Verification items for this drawing (mm, ordinates from the low corner). Give positions to 0.01 mm unless a question says otherwise; leave off trailing zeros. Write each loop counter-clockwise with the first axis right and the second up, starting at its lowest first coordinate (ties: lowest second). Pieces come first, ordered by that corner, then holes. Notation, with made-up numbers: (34.5, 43) -> (82.5, 43) arc R30 cw to (82.5, 70) -> close; hole circle Ø2 at (-21.5, 7). An arc over 180 degrees is marked (long way). Answer as a JSON object with one key per item and string values.
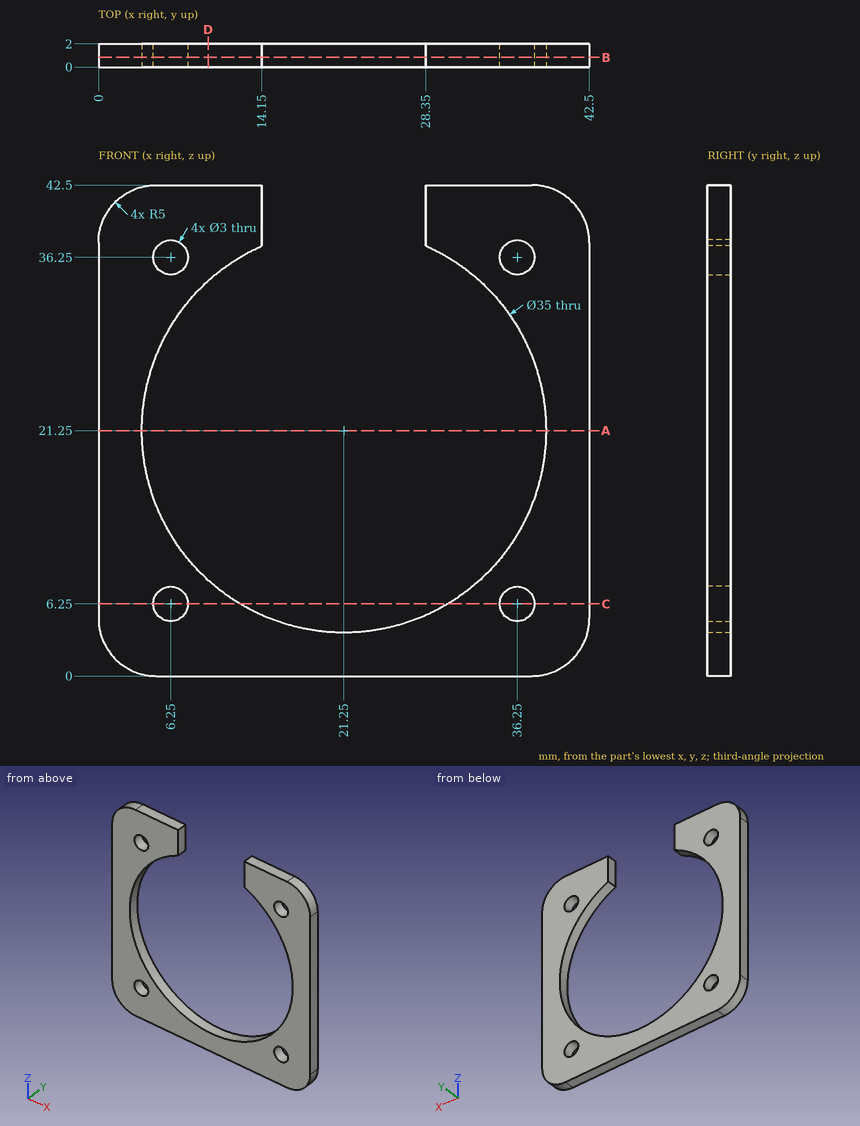
1. Sectioned sample at C-C, the plane z = 6.25. Enter the section's corners in (x, y).
Determined:
{"outline": "(0, 0) -> (4.75, 0) -> (4.75, 2) -> (0, 2) -> close; (7.75, 0) -> (12.24, 0) -> (12.24, 2) -> (7.75, 2) -> close; (30.26, 0) -> (34.75, 0) -> (34.75, 2) -> (30.26, 2) -> close; (37.75, 0) -> (42.5, 0) -> (42.5, 2) -> (37.75, 2) -> close"}
2. Go/stop test with flat-tipped pins: P1, Ø1, axis at y = 1.5, z = 39.5, coming from the +X side; P2, Ø1, axis at x = 17.5, y = 1, coming from the +Z side; P3, Ø1, axis at y = 1, z = 40.5, coming from the -X side. Record where each tip stops, or that it passes through.
Determined:
{"P1": "x = 42.27", "P2": "z = 4.27", "P3": "x = 0.67"}
3. Sectioned sample at A-A, the plane z = 21.25. Enter the section's corners in (x, y), plus the area to 3 significant figures.
Determined:
{"outline": "(0, 0) -> (3.75, 0) -> (3.75, 2) -> (0, 2) -> close; (38.75, 0) -> (42.5, 0) -> (42.5, 2) -> (38.75, 2) -> close", "area": "15.0 mm^2"}
4. Sectioned sample at B-B, the plane y = 0.85. Enter the section's corners in (x, z) (3 decimals).
Determined:
{"outline": "(0, 5) arc R5 ccw to (5, 0) -> (37.5, 0) arc R5 ccw to (42.5, 5) -> (42.5, 37.5) arc R5 ccw to (37.5, 42.5) -> (28.35, 42.5) -> (28.35, 37.245) arc R17.5 cw (long way) to (14.15, 37.245) -> (14.15, 42.5) -> (5, 42.5) arc R5 ccw to (0, 37.5) -> close; hole circle Ø3 at (6.25, 6.25); hole circle Ø3 at (6.25, 36.25); hole circle Ø3 at (36.25, 6.25); hole circle Ø3 at (36.25, 36.25)"}
5. Scan lines: L1, parallel to X at y = 0.4, z = 6.25; L2, parallel to X at y = 0.3, z = 21; L3, parallel to X at y = 1, z = 10.5. Record each from-to range of solid material in increasing order. Write a range as [from, to].
Determined:
{"L1": "[0, 4.75], [7.75, 12.24], [30.26, 34.75], [37.75, 42.5]", "L2": "[0, 3.75], [38.75, 42.5]", "L3": "[0, 7.44], [35.06, 42.5]"}
6. Sectioned sample at D-D, the plane x = 9.5. Enter the section's corners in (y, z).
Determined:
{"outline": "(0, 0) -> (2, 0) -> (2, 8.28) -> (0, 8.28) -> close; (0, 34.22) -> (2, 34.22) -> (2, 42.5) -> (0, 42.5) -> close"}
